Input: part model. Units: mm. Frame: model coordinates. Face numbers are marked on the shaded views. A direction names the side the tool comes from. Coordinates: 2 decimals unless noted, no trailing zeros. Loops run counter-clockwise (first coordinate to the right, second up) from the corner with the lowest first, then second, coordinate; pieces in that order, holes last. Notation, with made-up numbers: (-21.75, -39) -> (-10.75, -39) arc R19 cw to (-10.75, -26) -> close; hole circle Ø2 at (54.5, 35.25). An arc over 180 degrees is marked (long way). Answer as a JSON object with one key per item and string values.
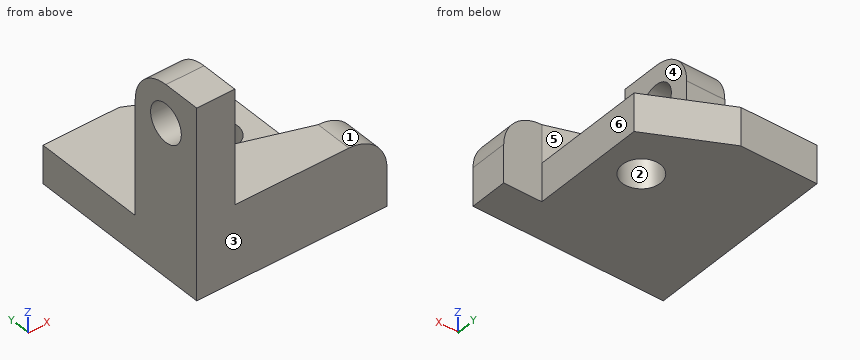
from build123d import *

# Parameters (mm, degrees)
EXTRUDE_1_DEPTH     = 5
SKETCH_1_3_W        = 20
SKETCH_1_3_H        = 5
EXTRUDE_2_DEPTH     = 10
SKETCH_1_4_W        = 20
SKETCH_1_4_H        = 5
EXTRUDE_3_DEPTH     = 25
SKETCH_2_R          = 2.5
CUT_EXTRUDE_1_DEPTH = 25
CUT_EXTRUDE_2_DEPTH = 5
SKETCH_4_R          = 2.5
EXTRUDE_4_DEPTH     = 5
SCALE_1_SCALE       = 0.2


with BuildPart() as part:
    # 草圖1 → 填料-伸長1 (new body)
    with BuildSketch(Plane(origin=(0, 0, 0), x_dir=(1, 0, 0), z_dir=(0, 1, 0))):
        with BuildLine():
            Line((20, 10), (20, 5))
            Line((20, 5), (20, 0))
            ThreePointArc((20, 0), (23.535533906, 1.464466094), (25, 5))
            Line((25, 5), (25, 10))
            Line((25, 10), (20, 10))
        make_face()
    extrude(amount=EXTRUDE_1_DEPTH)

    # 草圖1<3> → 填料-伸長2 (add)
    with BuildSketch(Plane(origin=(0, 0, 0), x_dir=(1, 0, 0), z_dir=(0, 1, 0))):
        with Locations((10, 2.5)):
            Rectangle(SKETCH_1_3_W, SKETCH_1_3_H)
    extrude(amount=EXTRUDE_2_DEPTH)

    # 草圖1<4> → 填料-伸長3 (add)
    with BuildSketch(Plane(origin=(0, 0, 0), x_dir=(1, 0, 0), z_dir=(0, 1, 0))):
        with Locations((10, 7.5)):
            Rectangle(SKETCH_1_4_W, SKETCH_1_4_H)
    extrude(amount=EXTRUDE_3_DEPTH)

    # 草圖2 → 除料-伸長1 (cut)
    with BuildSketch(Plane.XY.offset(-5)):
        with Locations((15, 15)):
            Circle(SKETCH_2_R)
        Polygon((10, 25), (20, 20), (20, 25), align=None)
    extrude(amount=-CUT_EXTRUDE_1_DEPTH, mode=Mode.SUBTRACT)

    # 草圖3 → 除料-伸長2 (cut)
    with BuildSketch(Plane.XY):
        Polygon((20, 5), (5, 10), (20, 10), align=None)
    extrude(amount=-CUT_EXTRUDE_2_DEPTH, mode=Mode.SUBTRACT)

    # 草圖4 → 填料-伸長4 (add)
    with BuildSketch(Plane(origin=(0, 0, 0), x_dir=(0, 0, -1), z_dir=(1, 0, 0))):
        with BuildLine():
            Line((0, 10), (-10, 10))
            ThreePointArc((-10, 10), (-13.535533906, 8.535533906), (-15, 5))
            Line((-15, 5), (-15, 0))
            Line((-15, 0), (0, 0))
            Line((0, 0), (0, 10))
        make_face()
        with Locations((-10, 5)):
            Circle(SKETCH_4_R, mode=Mode.SUBTRACT)
    extrude(amount=EXTRUDE_4_DEPTH)


with BuildPart() as part_1:
    # 縮放比例1: scaled about (8.934190185, 8.603677977, -4.077878453)
    add(part.part.scale(SCALE_1_SCALE).moved(Location((7.147352148, 6.882942382, -3.262302762))))


solid = part_1.part
1. Section query D-D (x = 10.45). Return loops of the section in (y, z).
Reply:
{"outline": "(6.88, -5.26) -> (9.48, -5.26) -> (9.48, -4.26) -> (8.12, -4.26) -> (8.12, -3.26) -> (6.88, -3.26) -> close; (10.28, -5.26) -> (11.23, -5.26) -> (11.23, -4.26) -> (10.28, -4.26) -> close"}
2. Mould query, pull axis X, two halves, no side actions, for the marked faces 1, 2 and 3. Classes: pulls with the +X half, pulls with the -X half, needs draft (parallel to the pull), parting line crosses it, or undercut.
Reply:
{"face 1": "pulls with the +X half", "face 2": "undercut", "face 3": "needs draft"}
3. Section query B-B (z = -1). Return loops of the section in (x, y).
Reply:
{"outline": "(7.15, 6.88) -> (8.15, 6.88) -> (8.15, 7.46) -> (7.15, 7.46) -> close; (7.15, 8.31) -> (8.15, 8.31) -> (8.15, 8.85) -> (7.15, 8.85) -> close"}
4. Section query A-A (x = 9.8). Return loops of the section in (y, z), plus the area to 3 significant figures.
Reply:
{"outline": "(6.88, -5.26) -> (9.52, -5.26) -> (9.52, -4.26) -> (8.33, -4.26) -> (8.33, -3.26) -> (6.88, -3.26) -> close; (10.24, -5.26) -> (11.56, -5.26) -> (11.56, -4.26) -> (10.24, -4.26) -> close", "area": "5.40 mm2"}
5. Access query for the marked faces 4, 5 and 6. Directions: +Z, -Z, +X, -X, +Y, -Y. A direction counts if a zero-diameter tool reaches every point of the face in a straight line with its end or side. Return the directions, or none.
Reply:
{"face 4": "+Z, +X, +Y, -Y", "face 5": "+Z, +X, +Y", "face 6": "+Z, -Z, +X, +Y"}
6. Pin query (flat end, axial travel): P1, Ø0.8, axis at x = 11.5, z = -4, coming from the +Y side; P2, Ø3, axis at x = 9, y = 9.5, coming from the +Z side; P3, Ø1.5, axis at x = 9, y = 9.5, coming from the +Z side. Return the tip coordinate at first contact, or that it passes through.
Reply:
{"P1": "stops at y = 7.9", "P2": "stops at z = -0.34", "P3": "stops at z = -4.26"}
7. Section query C-C (y = 8.2). Return loops of the section in (x, z).
Reply:
{"outline": "(7.15, -5.26) -> (11.15, -5.26) -> (11.15, -4.26) -> (10.2, -4.26) -> (10.2, -3.26) -> (8.15, -3.26) -> (8.15, -1.65) -> (7.15, -1.65) -> close; (7.15, -0.88) -> (8.15, -0.88) -> (8.15, -0.31) -> (7.15, -0.31) -> close"}
8. Line query: line 1 along Z through (x, y) = (7.4, 10.8); line 2 along Z through (x, y) = (9.8, 7.5); line 3 along Y through (x, z) = (11.3, -4.45). Output: solid intervals per line, ascending.
Reply:
{"line 1": "z = -5.26 to -4.26", "line 2": "z = -5.26 to -3.26", "line 3": "y = 6.88 to 7.88"}
